Can you work these out from the model? Positions are in its coordinate system, mm. A direction names the side the tool comes from. Round coordinates to 2 decimals unless told otherwise and drop trailing zeros. Write each loop counter-clockwise with the first axis right and the second up, starting at its lowest first coordinate (ties: lowest second). Pieces come first, ordered by that corner, then holes. Notation, with made-up numbers: M 3.25,-34.5 L 57.25,-34.5 A13 ccw 57.25,-25.5 Z; hole C -25.75,-15.5 d4. An arc over 180 degrees is marked long. Answer as a JSON object with one key per item and string values. Group by question number.
1) Please list where these lines run through material, in increasing order: L1, parallel to Y at x = 5, z = 4.5; L2, parallel to X at y = 0.75, z = 2. Write a range as [from, to].
2) Suppose I cut it at C-C, the plane z = 2.25. Write out the boundary of the cut face in (x, y).
3) On a 3-axis mill with a long thin cutter (end or side, diameter ignored), from which of +Z, -Z, +X, -X, +Y, -Y can I reach the whole of each face in a straight line? I mean faces 4 (the flat face through (3, 1, 0)), 5 (the flat face through (6, 1.524, 2)). Say none if no direction works.
4) Suppose I cut it at B-B, the plane y = 5.75. Write out the boundary of the cut face in (x, z), and give its area (3 significant figures).
5) If we mould it in two halves opening along X, with no side actions, what happens to faces 1 (the flat face through (0, 4, 3)), 2 (the cylindrical face through (7.896, 0.773, 2.849)), 3 (the cylindrical face through (0.773, 6.352, 4.062))? For each: +X half, -X half, draft (parallel to the pull), parting line (faces both ways), or undercut.
6) Suppose I cut it at A-A, the plane x = 6. Write out the boundary of the cut face in (y, z).
7) I'm going to push flat-ended pins straight in: pin 1 Ø3 at (x, y) = (8.5, 5) entering from -Z; pin 2 Ø3 at (y, z) = (4.5, 4.5) entering from +X. Where does each tip first touch, or does it pass through?
8) Suppose I cut it at D-D, the plane z = 4.75. Write out the boundary of the cut face in (x, y).
Autodesk Inventor part; units mm, degrees
ref_plane "YZ Plane" through (0, 0, 0) normal (1, 0, 0) x (0, 1, 0)
ref_plane "XZ Plane" through (0, 0, 0) normal (0, 1, 0) x (-1, 0, 0)
ref_plane "XY Plane" through (0, 0, 0) normal (0, 0, 1) x (1, 0, 0)
sketch "Sketch2" plane through (0, 0, 0) normal (0, 0, 1) x (1, 0, 0)
  line L0 (0, 8.763) -> (1.524, 8.763)
  line L1 (1.524, 8.763) -> (1.524, 1.524)
  line L2 (1.524, 1.524) -> (0, 1.524)
  line L3 (0, 1.524) -> (0, 8.763)
  line L4 (1.524, 1.524) -> (9.9822, 1.524)
  line L5 (9.9822, 1.524) -> (9.9822, 0)
  line L6 (9.9822, 0) -> (1.524, 0)
  line L7 (1.524, 0) -> (1.524, 1.524)
  arc A0 (0, 1.524) -> (1.524, 0) centre (1.524, 1.524) ccw
  point P0 (0, 0)
  dimension "d9" = 1.524
  dimension "d10" = 7.239
  dimension "d11" = 8.4582
extrude "Extrusion2" add sketch "Sketch2" along normal blind 6.4008
fillet "Fillet2" radius 0.508 4 edges at (0.762, 8.763, 6.4008) (0.762, 8.763, 0) (9.9822, 0.762, 6.4008) (9.9822, 0.762, 0)
sketch "Sketch3" plane through (1.524, 1.524, 6.4008) normal (0, 1, 0) x (1, 0, 0)
  circle A0 centre (5.2578, 3.2004) radius 1.1684
  line L0 (8.4582, 5.8928) -> (8.4582, 0.508)
  line L1 (7.9502, 0) -> (0, 0)
  point P0 (-1.524, 6.4008)
  point P1 (8.4582, 3.2004)
  dimension "d15" = 3.2004
  dimension "d16" = 3.2004
  dimension "d17" = 2.3368
extrude "Extrusion3" cut sketch "Sketch3" against normal through all
sketch "Sketch4" plane through (1.524, 1.524, 6.4008) normal (1, 0, 0) x (0, 0, -1)
  circle A0 centre (3.2004, 4.0386) radius 1.1684
  line L0 (5.8928, 7.239) -> (0.508, 7.239)
  line L1 (6.4008, 0) -> (6.4008, 6.731)
  point P0 (6.4008, -1.524)
  point P1 (3.2004, 7.239)
  dimension "d20" = 3.2004
  dimension "d21" = 3.2004
  dimension "d22" = 2.3368
extrude "Extrusion4" cut sketch "Sketch4" against normal through all
equation "\"d15\" = d16"
equation "\"d21\" = d20"
properties part number "elbow"
Results:
{
 "1": {"L1": "[0, 1.52]", "L2": "[0.21, 9.98]"},
 "2": {"outline": "M 0,1.52 A1.52 ccw 1.52,0 L 6.1,0 L 6.1,1.52 L 1.52,1.52 L 1.52,4.88 L 0,4.88 Z; M 0,6.24 L 1.52,6.24 L 1.52,8.76 L 0,8.76 Z; M 7.46,0 L 9.98,0 L 9.98,1.52 L 7.46,1.52 Z"},
 "3": {"face 4": "-Z, +X, -X, +Y, -Y", "face 5": "+Z, -Z, +X, +Y"},
 "4": {"outline": "M 0,0 L 1.52,0 L 1.52,2.05 L 0,2.05 Z; M 0,4.35 L 1.52,4.35 L 1.52,6.4 L 0,6.4 Z", "area": "6.24 mm^2"},
 "5": {"face 1": "-X half", "face 2": "undercut", "face 3": "draft"},
 "6": {"outline": "M 0,0 L 1.52,0 L 1.52,2.33 L 0,2.33 Z; M 0,4.07 L 1.52,4.07 L 1.52,6.4 L 0,6.4 Z"},
 "7": {"pin 1": "through", "pin 2": "x = 1.52"},
 "8": {"outline": "M 0,1.52 A1.52 ccw 1.52,0 L 9.98,0 L 9.98,1.52 L 1.52,1.52 L 1.52,8.76 L 0,8.76 Z"}
}
